Model file for the job. Use its own axes, mm. A direction names the side the tool comes from. Give positions to 0.01 mm unless a question says otherwise; leave off trailing zeros. Order: outer loops, then holes, each group sorted by start corner. A loop starts at its lowest first (then second) coordinate and runs counter-clockwise, first axis right, second up. Notation, with made-up numbers: M -7,-22 L 27,-22 A14 ccw 27,-8 Z; hole C 2,63 d4. An arc over 180 degrees is marked long. Return JSON: item names as keys, results as strings. Group by question number.
1. 3-axis set-ups, long thin cutter, end or side, ignore diameter. For faces 4 (the face through (0, 7, -25)), 5 (the face through (29.73, 0.49, -13.52)): which of +Z, -Z, +X, -X, +Y, -Y reach the whole face in a straight line?
2. Two-plate mould, pull along Z, no slides. Class faces 1 (the face through (-24, 6.34, 0.34)), 2 (the face through (29.77, 0.49, 13.48)), 3 (the face through (-23.964, 5.792, -24.493)): released by +Z, released by -Z, zero draft, split by the parting line, or undercut.
3. Slice it at B-B on x = 21. List the corners of the cut face in (y, z), then the cut area to 3 significant figures.
4. Slice it at C-C on y = 3.5. List the corners of the cut face in (x, z).
5. Pin check, flat tips, straight feed: pin 1 (8 mm diameter, centred on x = 26, y = 9, fed in from +Z); pin 2 (1 mm diameter, centred on x = -15.5, z = 12.5, fed in from +Y); pin 3 (6 mm diameter, centred on x = -1.5, z = -11.5, fed in from -Y). Stop position of each tip, or through.
6. Slice it at A-A on z = -20. List the corners of the cut face in (x, y), then the cut area to 3 significant figures.
7. Slice it at D-D on z = -7.5. List the corners of the cut face in (x, y), then the cut area to 3 significant figures.
8. Wall check: probe 1 along Y at (x, z) = (-16.5, -21); probe 2 along X at (y, z) = (20.5, 2.5); probe 3 along X at (y, z) = (11, -0.5). Give the ranges that are in metal, low to high. Write a range as [from, to].
from build123d import *

# Parameters (mm, degrees)
BOSS_EXTRUDE1_DEPTH   = 1
BOSS_EXTRUDE1_2_DEPTH = 1
BOSS_EXTRUDE2_DEPTH   = 50
CHAMFER1_SIZE         = 1


with BuildPart() as part:
    # Sketch1 → Boss-Extrude1 (new body)
    with BuildSketch(Plane(origin=(0, 0, 0), x_dir=(1, 0, 0), z_dir=(0, 1, 0))):
        Polygon((-28.25, 25), (-28.25, 15), (-31.25, 12), (-31.25, -12), (-28.25, -15), (-28.25, -25), (-33.25, -25), (-33.25, 25), align=None)
    extrude(amount=BOSS_EXTRUDE1_DEPTH)



with BuildPart() as body_2:
    # Sketch1 → Boss-Extrude1 2 (new body)
    with BuildSketch(Plane(origin=(0, 0, 0), x_dir=(1, 0, 0), z_dir=(0, 1, 0))):
        Polygon((33.25, 25), (28.25, 25), (28.25, 15), (31.25, 12), (31.25, -12), (28.25, -15), (28.25, -25), (33.25, -25), align=None)
    extrude(amount=BOSS_EXTRUDE1_2_DEPTH)


with BuildPart() as part_1:
    add(part.part)

    add(body_2.part)  # Boss-Extrude2 merges body 2
    # Sketch2 → Boss-Extrude2 (add)
    with BuildSketch(Plane.XY.offset(25)):
        with BuildLine():
            Line((-33.25, 1), (33.25, 1))
            Line((33.25, 1), (15, 11.536642413))
            ThreePointArc((15, 11.536642413), (7.060428276, 17.552838357), (0.853658537, 25.344335145))
            ThreePointArc((0.853658537, 25.344335145), (0, 25.82350206), (-0.853658537, 25.344335145))
            ThreePointArc((-0.853658537, 25.344335145), (-7.060428276, 17.552838357), (-15, 11.536642413))
            Line((-15, 11.536642413), (-33.25, 1))
        make_face()
    extrude(amount=-BOSS_EXTRUDE2_DEPTH)

    # Chamfer1
    chamfer1_edges = [part_1.edges().sort_by_distance(p)[0] for p in [
        (24.125, 6.268321206, -25),
        (24.125, 6.268321206, 25),
        (7.060428276, 17.552838357, -25),
        (7.060428276, 17.552838357, 25),
        (0, 25.82350206, -25),
        (0, 25.82350206, 25),
        (-24.125, 6.268321206, -25),
        (-24.125, 6.268321206, 25),
        (-7.060428276, 17.552838357, -25),
        (-7.060428276, 17.552838357, 25),
    ]]
    chamfer(chamfer1_edges, length=CHAMFER1_SIZE)


solid = part_1.part
Result:
{
 "1": {"face 4": "-Z, +X, -X, +Y, -Y", "face 5": "-Y"},
 "2": {"face 1": "zero draft", "face 2": "undercut", "face 3": "released by -Z"},
 "3": {"outline": "M 1,-25 L 6.92,-25 L 8.07,-24 L 8.07,24 L 6.92,25 L 1,25 Z", "area": "352 mm2"},
 "4": {"outline": "M -28.92,-24 L -26.92,-25 L 26.92,-25 L 28.92,-24 L 28.92,24 L 26.92,25 L -26.92,25 L -28.92,24 Z"},
 "5": {"pin 1": "stops at z = 24.7", "pin 2": "stops at y = 11.54", "pin 3": "stops at y = 1"},
 "6": {"outline": "M -33.25,0 L -28.25,0 L -28.25,1 L 28.25,1 L 28.25,0 L 33.25,0 L 33.25,1 L 15,11.54 A40 cw 0.85,25.34 A1 ccw -0.85,25.34 A40 cw -15,11.54 L -33.25,1 Z", "area": "705 mm2"},
 "7": {"outline": "M -33.25,0 L -31.25,0 L -31.25,1 L 31.25,1 L 31.25,0 L 33.25,0 L 33.25,1 L 15,11.54 A40 cw 0.85,25.34 A1 ccw -0.85,25.34 A40 cw -15,11.54 L -33.25,1 Z", "area": "699 mm2"},
 "8": {"probe 1": "y = [1, 10.67]", "probe 2": "x = [-4.33, 4.33]", "probe 3": "x = [-15.93, 15.93]"}
}
